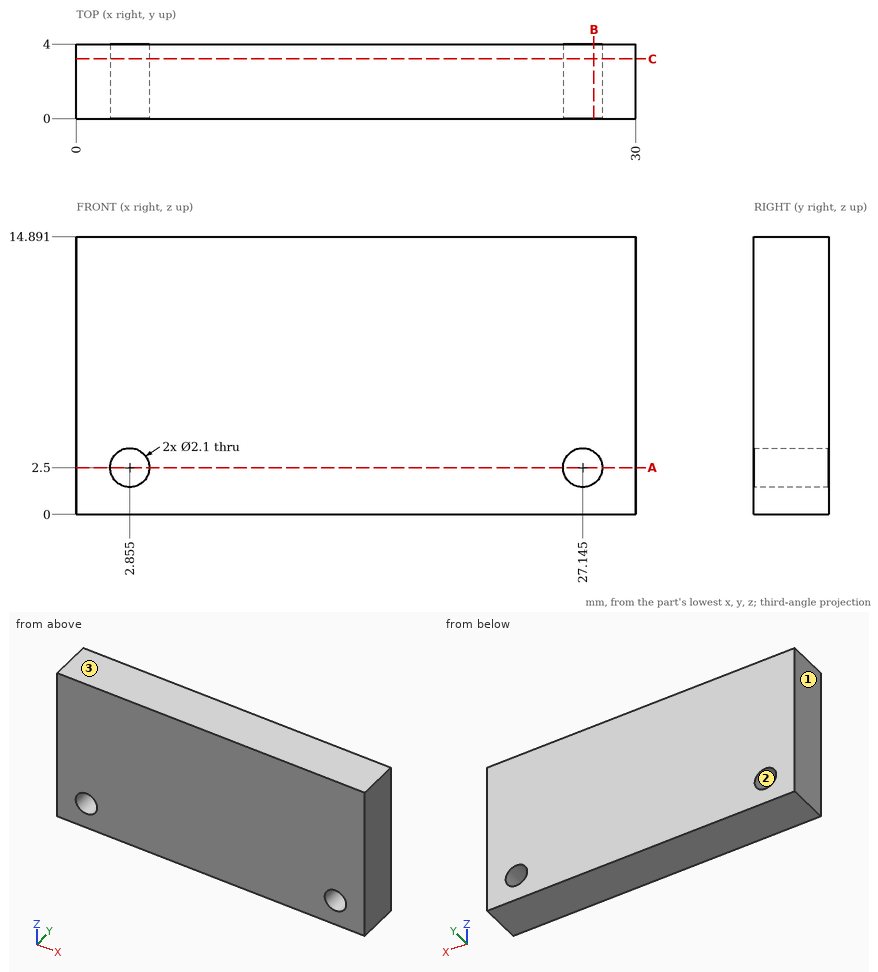
Job drawing, mm, ordinate dimensions from the low corner. One solid piece. Round coordinates to 2 decimals unless told otherwise and drop trailing zeros. Write each loop counter-clockwise with the first axis right and the second up, starting at its lowest first coordinate (ties: lowest second). Pieces come first, ordered by that corner, then holes.
1) Drill centre lines: probe 1 along X at (y, z) = (2.1, 2.5) (3 decimals); probe 2 along X at (y, z) = (1, 3.25); probe 3 along Z at (x, y) = (2.25, 1.5). Where is each one in solid material? Low to high.
2) Band-saw the part on C-C, the plane y = 3.2. List the corners of the cut face in (x, z) (3 decimals), and give its area (3 significant figures).
3) Mould opens along X. For the marked faces 1, 2 and 3 say: +X half, -X half, draft (parallel to the pull), parting line (faces both ways), or undercut.
4) Band-saw the part on A-A, the plane z = 2.5. List the corners of the cut face in (x, y) (3 decimals), and give its area (3 significant figures).
5) Band-saw the part on B-B, the plane x = 27.75. List the corners of the cut face in (y, z), and give its area (3 significant figures).
Ans:
1. probe 1: x = 0 to 1.805, 3.905 to 26.095, 28.195 to 30
1. probe 2: x = 0 to 2.12, 3.59 to 26.41, 27.88 to 30
1. probe 3: z = 0 to 1.64, 3.36 to 14.89
2. outline: (0, 0) - (30, 0) - (30, 14.891) - (0, 14.891) - close; hole circle Ø2.1 at (2.855, 2.5); hole circle Ø2.1 at (27.145, 2.5)
2. area: 440 mm2
3. face 1: -X half
3. face 2: undercut
3. face 3: draft
4. outline: (0, 0) - (1.805, 0) - (1.805, 4) - (0, 4) - close; (3.905, 0) - (26.095, 0) - (26.095, 4) - (3.905, 4) - close; (28.195, 0) - (30, 0) - (30, 4) - (28.195, 4) - close
4. area: 103 mm2
5. outline: (0, 0) - (4, 0) - (4, 1.64) - (0, 1.64) - close; (0, 3.36) - (4, 3.36) - (4, 14.89) - (0, 14.89) - close
5. area: 52.7 mm2
